Geometry: final body of the model. Coordinates: model frame, mm. Face numbers are marked on the shaded views. A direction names the side the tool comes from. Coordinates: 2 decimals unless noted, no trailing zeros. Order: outer loops, then holes, each group sorted by start corner. A loop starts at its lowest first (then second) coordinate and runs counter-clockwise, first axis right, second up. Notation, with made-up numbers: M 11,-34 L 58,-34 A24 cw 58,-1 Z; hole C 61,66.25 d1. An arc over 180 degrees is marked long. Write item = value, one per line. Start each with the question number.
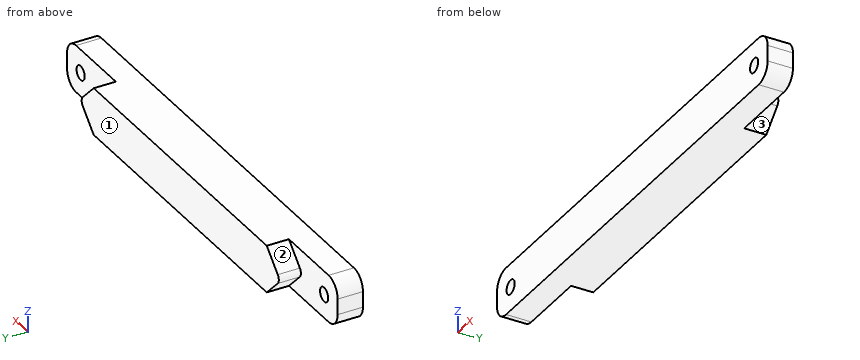
```python
from build123d import *

# Parameters (mm, degrees)
SKETCH1_W            = 150
SKETCH1_H            = 15
BOSS_EXTRUDE1_DEPTH  = 15
SKETCH2_W            = 16
SKETCH2_H            = 15
CUT_EXTRUDE1_DEPTH   = 7
SKETCH3_R            = 2.25
CUT_EXTRUDE2_DEPTH   = 8
FILLET1_R            = 5
CUT_EXTRUDE3_DEPTH   = 7
FILLET2_R            = 2
FILLET2_OF_MIRROR2_R = 2


with BuildPart() as part:
    # Sketch1 → Boss-Extrude1 (new body)
    with BuildSketch(Plane(origin=(0, 0, 0), x_dir=(1, 0, 0), z_dir=(0, 1, 0))):
        with Locations((75, 7.5)):
            Rectangle(SKETCH1_W, SKETCH1_H)
    extrude(amount=BOSS_EXTRUDE1_DEPTH)

    # Sketch2 → Cut-Extrude1 (cut)
    with BuildSketch(Plane(origin=(0, 15, 0), x_dir=(1, 0, 0), z_dir=(0, 1, 0))):
        with Locations((8, 7.5)):
            Rectangle(SKETCH2_W, SKETCH2_H)
    cut_extrude1 = extrude(amount=-CUT_EXTRUDE1_DEPTH, mode=Mode.SUBTRACT)

    # Sketch3 → Cut-Extrude2 (cut)
    with BuildSketch(Plane(origin=(0, 8, 0), x_dir=(1, 0, 0), z_dir=(0, 1, 0))):
        with Locations((7.5, 7.5)):
            Circle(SKETCH3_R)
    cut_extrude2 = extrude(amount=-CUT_EXTRUDE2_DEPTH, mode=Mode.SUBTRACT)

    # Mirror1: Cut-Extrude1, Cut-Extrude2 across plane
    add(cut_extrude1.mirror(Plane(origin=(75, 0, 0), x_dir=(0, 0, 1), z_dir=(1, 0, 0))), mode=Mode.SUBTRACT)
    add(cut_extrude2.mirror(Plane(origin=(75, 0, 0), x_dir=(0, 0, 1), z_dir=(1, 0, 0))), mode=Mode.SUBTRACT)

    # Fillet1
    fillet1_edges = [part.edges().sort_by_distance(p)[0] for p in [
        (0, 4, -15),
        (0, 4, 0),
        (150, 4, -15),
        (150, 4, 0),
    ]]
    fillet(fillet1_edges, radius=FILLET1_R)

    # Sketch4 → Cut-Extrude3 (cut)
    with BuildSketch(Plane(origin=(0, 15, 0), x_dir=(1, 0, 0), z_dir=(0, 1, 0))):
        Polygon((19.52081528, 7.5), (16, 11.02081528), (16, 0), (27.02081528, 0), align=None)
        Polygon((16, 15), (16, 11.02081528), (19.52081528, 7.5), (27.02081528, 15), align=None)
    cut_extrude3 = extrude(amount=-CUT_EXTRUDE3_DEPTH, mode=Mode.SUBTRACT)

    # Fillet2
    fillet2_edges = [part.edges().sort_by_distance(p)[0] for p in [
        (19.52081528, 11.5, -7.5),
    ]]
    fillet(fillet2_edges, radius=FILLET2_R)

    # Mirror2: Cut-Extrude3 across plane
    add(cut_extrude3.mirror(Plane(origin=(75, 0, 0), x_dir=(0, 0, 1), z_dir=(1, 0, 0))), mode=Mode.SUBTRACT)

    # Fillet2 of Mirror2
    fillet2_of_mirror2_edges = [part.edges().sort_by_distance(p)[0] for p in [
        (130.47918472, 11.5, -7.5),
    ]]
    fillet(fillet2_of_mirror2_edges, radius=FILLET2_OF_MIRROR2_R)


solid = part.part
```
Item 1: Section query D-D on y = 12.5. Output: boundary loops of the cut face in (x, z), and give its area (3 significant figures).
Item 2: Section query B-B on x = 7.5. Output: boundary loops of the cut face in (y, z).
Item 3: First-contact query: pin 1 (5 mm diameter, centred on x = 61, z = -10.5, fed in from -Y); pin 2 (3 mm diameter, centred on y = 11.5, z = -7, fed in from -X). Flat tips, straight axial feed; report the tip coordinate or a pass-through.
Item 4: Section query C-C on y = 1.75. Output: boundary loops of the cut face in (x, z).
Item 5: Material intervals for probe 1 along X at (y, z) = (6.5, -7.5); probe 2 along Z at (x, y) = (142.5, 4); probe 3 along X at (y, z) = (6.5, -6.25), sorted ascending. Write a range as [from, to].
Item 6: Reachability of the marked faces 1, 2 and 3 from +Z, -Z, +X, -X, +Y, -Y: full face, straight path, thin tool, end or side. Return the list, or none.
Item 7: Section query A-A on z = -7.5. Output: boundary loops of the cut face in (x, y).
Ans:
q1.outline = M 20.94,-8.91 L 27.02,-15 L 122.98,-15 L 129.06,-8.91 A2 ccw 129.06,-6.09 L 122.98,0 L 27.02,0 L 20.94,-6.09 A2 ccw Z
q1.area = 1,550 mm^2
q2.outline = M 0,-15 L 8,-15 L 8,-9.75 L 0,-9.75 Z; M 0,-5.25 L 8,-5.25 L 8,0 L 0,0 Z
q3.pin_1 = 0
q3.pin_2 = 20.35
q4.outline = M 0,-10 A5 ccw 5,-15 L 145,-15 A5 ccw 150,-10 L 150,-5 A5 ccw 145,0 L 5,0 A5 ccw 0,-5 Z; hole C 7.5,-7.5 d4.5; hole C 142.5,-7.5 d4.5
q5.probe_1 = [0, 5.25], [9.75, 140.25], [144.75, 150]
q5.probe_2 = [-15, -9.75], [-5.25, 0]
q5.probe_3 = [0, 5.63], [9.37, 140.63], [144.37, 150]
q6.face_1 = +Z, -Z, +X, -X, +Y
q6.face_2 = +Z, -X, +Y
q6.face_3 = -Z, +X, +Y
q7.outline = M 0,0 L 5.25,0 L 5.25,8 L 0,8 Z; M 9.75,0 L 140.25,0 L 140.25,8 L 129.65,8 L 129.65,15 L 20.35,15 L 20.35,8 L 9.75,8 Z; M 144.75,0 L 150,0 L 150,8 L 144.75,8 Z
